from build123d import *

# Parameters (mm, degrees)
ESQUISSE1_R        = 2.1
BOSS_EXTRU_1_DEPTH = 125


with BuildPart() as part:
    # Esquisse1 → Boss.-Extru.1 (new, symmetric)
    with BuildSketch(Plane.XY):
        with BuildLine():
            Line((-20, 3.750660172), (-22.69, 3.750660172))
            Line((-22.69, 3.750660172), (-25.499339828, 6.56))
            Line((-25.499339828, 6.56), (-25.499339828, 8.2))
            Line((-25.499339828, 8.2), (-22.69, 8.2))
            Line((-22.69, 8.2), (-24.49, 10))
            Line((-24.49, 10), (-28.2, 10))
            ThreePointArc((-28.2, 10), (-29.472792206, 9.472792206), (-30, 8.2))
            Line((-30, 8.2), (-30, 4.49))
            Line((-30, 4.49), (-28.2, 2.69))
            Line((-28.2, 2.69), (-28.2, 5.499339828))
            Line((-28.2, 5.499339828), (-26.56, 5.499339828))
            Line((-26.56, 5.499339828), (-23.750660172, 2.69))
            Line((-23.750660172, 2.69), (-23.750660172, 0))
            Line((-23.750660172, 0), (-23.750660172, -2.69))
            Line((-23.750660172, -2.69), (-26.56, -5.499339828))
            Line((-26.56, -5.499339828), (-28.2, -5.499339828))
            Line((-28.2, -5.499339828), (-28.2, -2.69))
            Line((-28.2, -2.69), (-30, -4.49))
            Line((-30, -4.49), (-30, -8.2))
            ThreePointArc((-30, -8.2), (-29.472792206, -9.472792206), (-28.2, -10))
            Line((-28.2, -10), (-24.49, -10))
            Line((-24.49, -10), (-22.69, -8.2))
            Line((-22.69, -8.2), (-25.499339828, -8.2))
            Line((-25.499339828, -8.2), (-25.499339828, -6.56))
            Line((-25.499339828, -6.56), (-22.69, -3.750660172))
            Line((-22.69, -3.750660172), (-20, -3.750660172))
            Line((-20, -3.750660172), (-17.31, -3.750660172))
            Line((-17.31, -3.750660172), (-14.500660172, -6.56))
            Line((-14.500660172, -6.56), (-14.500660172, -8.2))
            Line((-14.500660172, -8.2), (-17.31, -8.2))
            Line((-17.31, -8.2), (-15.51, -10))
            Line((-15.51, -10), (-4.49, -10))
            Line((-4.49, -10), (-2.69, -8.2))
            Line((-2.69, -8.2), (-5.499339828, -8.2))
            Line((-5.499339828, -8.2), (-5.499339828, -6.56))
            Line((-5.499339828, -6.56), (-2.69, -3.750660172))
            Line((-2.69, -3.750660172), (2.69, -3.750660172))
            Line((2.69, -3.750660172), (5.499339828, -6.56))
            Line((5.499339828, -6.56), (5.499339828, -8.2))
            Line((5.499339828, -8.2), (2.69, -8.2))
            Line((2.69, -8.2), (4.49, -10))
            Line((4.49, -10), (15.51, -10))
            Line((15.51, -10), (17.31, -8.2))
            Line((17.31, -8.2), (14.500660172, -8.2))
            Line((14.500660172, -8.2), (14.500660172, -6.56))
            Line((14.500660172, -6.56), (17.31, -3.750660172))
            Line((17.31, -3.750660172), (20, -3.750660172))
            Line((20, -3.750660172), (22.69, -3.750660172))
            Line((22.69, -3.750660172), (25.499339828, -6.56))
            Line((25.499339828, -6.56), (25.499339828, -8.2))
            Line((25.499339828, -8.2), (22.69, -8.2))
            Line((22.69, -8.2), (24.49, -10))
            Line((24.49, -10), (28.2, -10))
            ThreePointArc((28.2, -10), (29.472792206, -9.472792206), (30, -8.2))
            Line((30, -8.2), (30, -4.49))
            Line((30, -4.49), (28.2, -2.69))
            Line((28.2, -2.69), (28.2, -5.499339828))
            Line((28.2, -5.499339828), (26.56, -5.499339828))
            Line((26.56, -5.499339828), (23.750660172, -2.69))
            Line((23.750660172, -2.69), (23.750660172, 0))
            Line((23.750660172, 0), (23.750660172, 2.69))
            Line((23.750660172, 2.69), (26.56, 5.499339828))
            Line((26.56, 5.499339828), (28.2, 5.499339828))
            Line((28.2, 5.499339828), (28.2, 2.69))
            Line((28.2, 2.69), (30, 4.49))
            Line((30, 4.49), (30, 8.2))
            ThreePointArc((30, 8.2), (29.472792206, 9.472792206), (28.2, 10))
            Line((28.2, 10), (24.49, 10))
            Line((24.49, 10), (22.69, 8.2))
            Line((22.69, 8.2), (25.499339828, 8.2))
            Line((25.499339828, 8.2), (25.499339828, 6.56))
            Line((25.499339828, 6.56), (22.69, 3.750660172))
            Line((22.69, 3.750660172), (20, 3.750660172))
            Line((20, 3.750660172), (17.31, 3.750660172))
            Line((17.31, 3.750660172), (14.500660172, 6.56))
            Line((14.500660172, 6.56), (14.500660172, 8.2))
            Line((14.500660172, 8.2), (17.31, 8.2))
            Line((17.31, 8.2), (15.51, 10))
            Line((15.51, 10), (4.49, 10))
            Line((4.49, 10), (2.69, 8.2))
            Line((2.69, 8.2), (5.499339828, 8.2))
            Line((5.499339828, 8.2), (5.499339828, 6.56))
            Line((5.499339828, 6.56), (2.69, 3.750660172))
            Line((2.69, 3.750660172), (-2.69, 3.750660172))
            Line((-2.69, 3.750660172), (-5.499339828, 6.56))
            Line((-5.499339828, 6.56), (-5.499339828, 8.2))
            Line((-5.499339828, 8.2), (-2.69, 8.2))
            Line((-2.69, 8.2), (-4.49, 10))
            Line((-4.49, 10), (-15.51, 10))
            Line((-15.51, 10), (-17.31, 8.2))
            Line((-17.31, 8.2), (-14.500660172, 8.2))
            Line((-14.500660172, 8.2), (-14.500660172, 6.56))
            Line((-14.500660172, 6.56), (-17.31, 3.750660172))
            Line((-17.31, 3.750660172), (-20, 3.750660172))
        make_face()
        Circle(ESQUISSE1_R, mode=Mode.SUBTRACT)
        with Locations((-20, 0)):
            Circle(ESQUISSE1_R, mode=Mode.SUBTRACT)
        with Locations((20, 0)):
            Circle(ESQUISSE1_R, mode=Mode.SUBTRACT)
        Polygon((-28.2, 8.2), (-28.2, 6.569339828), (-27.63, 6.569339828), (-26.569339828, 7.63), (-26.569339828, 8.2), align=None, mode=Mode.SUBTRACT)
        Polygon((-26.569339828, -7.63), (-27.63, -6.569339828), (-28.2, -6.569339828), (-28.2, -8.2), (-26.569339828, -8.2), align=None, mode=Mode.SUBTRACT)
        Polygon((-7.300660172, -8.2), (-7.300660172, -6.24), (-3.750660172, -2.69), (-3.750660172, 2.69), (-7.300660172, 6.24), (-7.300660172, 8.2), (-12.699339828, 8.2), (-12.699339828, 6.24), (-16.249339828, 2.69), (-16.249339828, -2.69), (-12.699339828, -6.24), (-12.699339828, -8.2), align=None, mode=Mode.SUBTRACT)
        Polygon((26.569339828, 8.2), (28.2, 8.2), (28.2, 6.569339828), (27.63, 6.569339828), (26.569339828, 7.63), align=None, mode=Mode.SUBTRACT)
        Polygon((26.569339828, -8.2), (26.569339828, -7.63), (27.63, -6.569339828), (28.2, -6.569339828), (28.2, -8.2), align=None, mode=Mode.SUBTRACT)
        Polygon((7.300660172, 8.2), (7.300660172, 6.24), (3.750660172, 2.69), (3.750660172, -2.69), (7.300660172, -6.24), (7.300660172, -8.2), (12.699339828, -8.2), (12.699339828, -6.24), (16.249339828, -2.69), (16.249339828, 2.69), (12.699339828, 6.24), (12.699339828, 8.2), align=None, mode=Mode.SUBTRACT)
    extrude(amount=BOSS_EXTRU_1_DEPTH, both=True)


solid = part.part
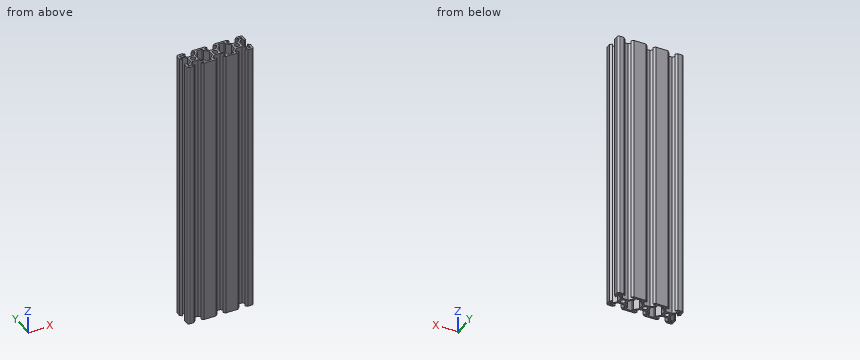
Input: part model. Units: mm. Frame: model coordinates. Round coordinates to 2 decimals unless told otherwise and drop trailing zeros. Loops run counter-clockwise (first coordinate to the right, second up) from the corner with the lowest first, then second, coordinate; pieces in that order, holes last. Notation, with made-up numbers: M -17,64 L 8,64 A24 cw 8,98 Z; hole C 45,22 d9. An arc over 180 degrees is marked long. Answer as CSV lines item,"result". Start each with the question number.
(1) Section C-C, the plane z = -71.5. State how many separate pieces and enclosed holes the cut face has, plus the area to 3 significant figures.
(2) Line query: line 1 (X direction, y = -2.25, z = 58.5); line 2 (Y direction, x = -11, z = 25); line 3 (X direction, y = 1.75, z = -24). Output: solid intervals per line, ascending. Write a range as [from, to].
(3) Section B-B, the plane y = 0. Output: boundary loops of the cut face in (x, z), plus the area to 3 significant figures.
(4) First-contact query: pin 1 (5 mm diameter, centred on x = -20, y = 0, fed in from -Z); pin 2 (3.5 mm diameter, centred on x = 0, y = 0, fed in from -Z); pin 3 (1.6 mm diameter, centred on x = -20.5, z = 29.5, fed in from +Y). Flat tips, straight axial feed; report the tip coordinate or a pass-through.
(5) Section A-A, the plane x = 20. Output: boundary loops of the cut face in (y, z).
Values found:
1,separate pieces,"1"
1,enclosed holes,"9"
1,area,"412 mm²"
2,line 1,"x = [-23.75, -16.25], [-3.75, 3.75], [16.25, 23.75]"
2,line 2,"y = [-10, -8.2], [8.2, 10]"
2,line 3,"x = [-23.75, -21.16], [-18.84, -16.25], [-3.75, -1.16], [1.16, 3.75], [16.25, 18.84], [21.16, 23.75]"
3,outline,"M -23.75,-125 L -22.1,-125 L -22.1,125 L -23.75,125 Z; M -17.9,-125 L -16.25,-125 L -16.25,125 L -17.9,125 Z; M -3.75,-125 L -2.1,-125 L -2.1,125 L -3.75,125 Z; M 2.1,-125 L 3.75,-125 L 3.75,125 L 2.1,125 Z; M 16.25,-125 L 17.9,-125 L 17.9,125 L 16.25,125 Z; M 22.1,-125 L 23.75,-125 L 23.75,125 L 22.1,125 Z"
3,area,"2,480 mm²"
4,pin 1,"stops at z = -125"
4,pin 2,"passes through"
4,pin 3,"stops at y = 3.75"
5,outline,"M -3.75,-125 L -2.1,-125 L -2.1,125 L -3.75,125 Z; M 2.1,-125 L 3.75,-125 L 3.75,125 L 2.1,125 Z"
